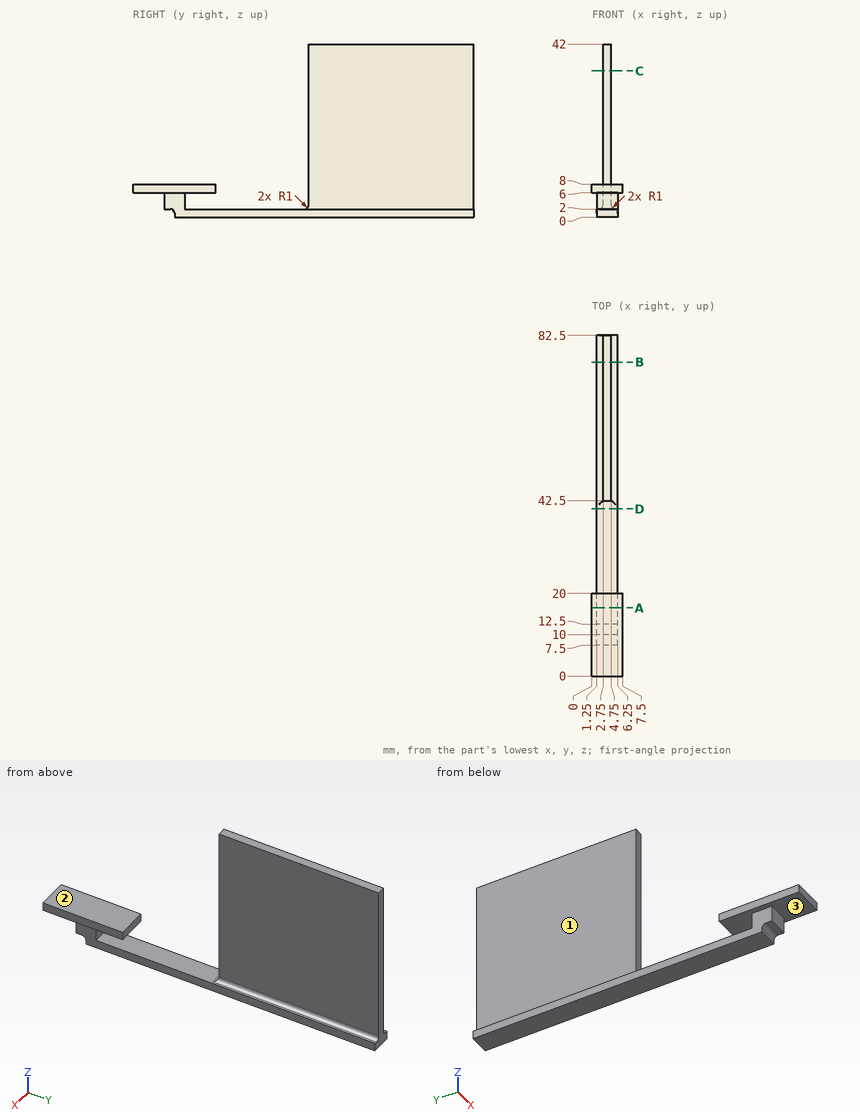
Print and shaded views of the part. All mm, measured from the part's lowest x, y and z. Round coordinates to 2 decimals unless told otherwise and drop trailing zeros. Loops run counter-clockwise (first coordinate to the right, second up) from the corner with the lowest first, then second, coordinate; pieces in that order, holes last. Notation, with made-up numbers: M 73.5,23.25 L 127.5,23.25 A16 ccw 127.5,34.25 Z; hole C 27,-35 d7. An arc over 180 degrees is marked long. One line per question, with ' | ' between items.
1) Band-saw the part on A-A (y = 16.5). Give the cut face in (x, z), then the cut area to 3 significant figures.
Solved:
outline: M 0,6 L 7.5,6 L 7.5,8 L 0,8 Z; M 1.25,0 L 6.25,0 L 6.25,2 L 1.25,2 Z | area: 25.0 mm²
2) Mould opens along Z. For the marked faces 1, 2 and 3 say: +Z half, -Z half, draft (parallel to the pull), parting line (faces both ways), or undercut.
Solved:
face 1: draft | face 2: +Z half | face 3: undercut
3) Band-saw the part on C-C (z = 35.5). Give the cut face in (x, y), then the cut area to 3 significant figures.
Solved:
outline: M 2.75,42.5 L 4.75,42.5 L 4.75,82.5 L 2.75,82.5 Z | area: 80.0 mm²
4) Drill centre lines: line 1 along Y through (x, z) = (3.75, 4); line 2 along Z through (x, y) = (1.75, 14.5); line 3 along X through (y, z) = (49, 32). Where is each one in solid material? Low to high.
Solved:
line 1: y = 7.5 to 12.5, 42.5 to 82.5 | line 2: z = 0 to 2, 6 to 8 | line 3: x = 2.75 to 4.75
5) Band-saw the part on B-B (y = 76). Give the cut face in (x, z), then the cut area to 3 significant figures.
Solved:
outline: M 1.25,0 L 6.25,0 L 6.25,2 L 5.75,2 A1 cw 4.75,3 L 4.75,42 L 2.75,42 L 2.75,3 A1 cw 1.75,2 L 1.25,2 Z | area: 90.4 mm²
6) Flat gauge pins, fed straight in: pin 1 (4 mm diameter, centred on y = 67.5, z = 5.5, fed in from -X); pin 2 (1.6 mm diameter, centred on x = 3, y = 8.5, fed in from -Z); pin 3 (6.5 mm diameter, centred on y = 28, z = 2, fed in from -X); pin 4 (1 mm diameter, centred on x = 2, y = 71, fed in from -Z). Where does each tip first touch, or does it go through?
Solved:
pin 1: stops at x = 2.75 | pin 2: stops at z = 1.95 | pin 3: stops at x = 1.25 | pin 4: stops at z = 0
7) Band-saw the part on D-D (y = 40.5). Give the cut face in (x, z).
Solved:
outline: M 1.25,0 L 6.25,0 L 6.25,2 L 1.25,2 Z
